Could you check a few things on this model? Use its own coordinates, in mm. Face numbers are marked on the shaded views. A direction names the side the tool comes from. Coordinates: 2 decimals unless noted, no trailing zeros. Loops run counter-clockwise (first coordinate to the right, second up) from the corner with the lowest first, then second, coordinate; pieces in that order, holes last.
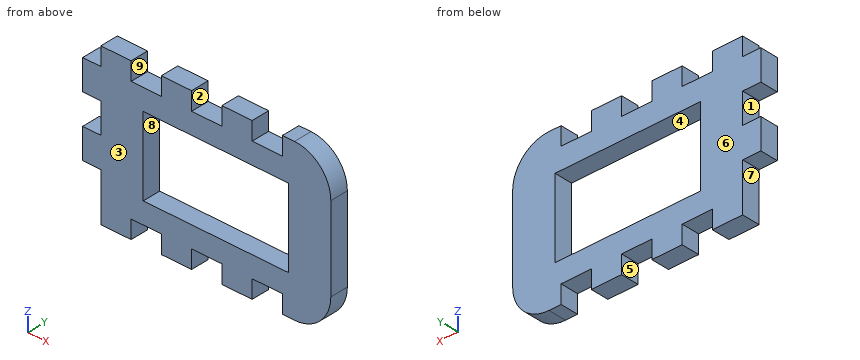
from build123d import *

# Parameters (mm, degrees)
SKETCH1_W           = 38
SKETCH1_H           = 26
BOSS_EXTRUDE1_DEPTH = 1.5
SKETCH2_W           = 24
SKETCH2_H           = 13
CUT_EXTRUDE1_DEPTH  = 3
SKETCH8_W           = 5
SKETCH8_H           = 3
BOSS_EXTRUDE2_DEPTH = 3
SKETCH9_W           = 5
SKETCH9_H           = 3
CUT_EXTRUDE2_DEPTH  = 3
FILLET1_R           = 6


with BuildPart() as part:
    # Sketch1 → Boss-Extrude1 (new body, symmetric)
    with BuildSketch(Plane(origin=(0, 0, 0), x_dir=(1, 0, 0), z_dir=(0, 1, 0))):
        Rectangle(SKETCH1_W, SKETCH1_H)
    extrude(amount=BOSS_EXTRUDE1_DEPTH, both=True)

    # Sketch2 → Cut-Extrude1 (cut)
    with BuildSketch(Plane.XZ.offset(1.5)):
        Rectangle(SKETCH2_W, SKETCH2_H)
    extrude(amount=-CUT_EXTRUDE1_DEPTH, mode=Mode.SUBTRACT)

    # Sketch8 → Boss-Extrude2 (add)
    with BuildSketch(Plane.ZY.offset(19)):
        with Locations((-2.5, 0)):
            Rectangle(SKETCH8_W, SKETCH8_H)
        with Locations((7.5, 0)):
            Rectangle(SKETCH8_W, SKETCH8_H)
    extrude(amount=BOSS_EXTRUDE2_DEPTH)

    # Sketch9 → Cut-Extrude2 (cut)
    with BuildSketch(Plane.XZ.offset(1.5)):
        with Locations((-11.5, -11.5)):
            Rectangle(SKETCH9_W, SKETCH9_H)
        with Locations((-11.5, 11.5)):
            Rectangle(SKETCH9_W, SKETCH9_H)
        with Locations((-1.5, -11.5)):
            Rectangle(SKETCH9_W, SKETCH9_H)
        with Locations((-1.5, 11.5)):
            Rectangle(SKETCH9_W, SKETCH9_H)
        with Locations((8.5, -11.5)):
            Rectangle(SKETCH9_W, SKETCH9_H)
        with Locations((8.5, 11.5)):
            Rectangle(SKETCH9_W, SKETCH9_H)
    extrude(amount=-CUT_EXTRUDE2_DEPTH, mode=Mode.SUBTRACT)

    # Fillet1
    fillet1_edges = [part.edges().sort_by_distance(p)[0] for p in [
        (19, 0, 13),
        (19, 0, -13),
    ]]
    fillet(fillet1_edges, radius=FILLET1_R)


solid = part.part
1) Imagine slicing it at A-A on z = 6. List the corners of the cut face in (x, y) for me.
2) For the marked faces 1, 2, 3, 4 and 5, which set-ups out of +Z, -Z, +X, -X, +Y, -Y let a thin tool reach every point of the face, with its end or its side?
3) If I drill on L1, parallel to X at y = 0.8, z = 1; L2, parallel to Z at x = -5, y = -0.1; L3, parallel to X at y = 0.1, z = -1.5, over which ranges is the centre line in solid material (lowest first)?
4) Will these pins go through, and if not, where does the flat tip stop? pin 1 (1 mm diameter, centred on y = -0.5, z = 8, fed in from +X); pin 2 (1.5 mm diameter, centred on y = 0.5, z = 3, fed in from -X); pin 3 (1.5 mm diameter, centred on y = 0, z = -11, fed in from +X).
5) We'd pull the mould along X, two halves only. Please class the marked faces 6, 7, 8 and 9: released by +X, released by -X, zero draft, split by the parting line, or undercut.
6) Imagine slicing it at B-B on x = 10. List the corners of the cut face in (y, z) for me.
Solved:
1. outline: (-22, -1.5) - (-12, -1.5) - (-12, 1.5) - (-22, 1.5) - close; (12, -1.5) - (19, -1.5) - (19, 1.5) - (12, 1.5) - close
2. face 1: -X, +Y, -Y
2. face 2: +Z, +Y, -Y
2. face 3: +Z, -Z, +X, -X, -Y
2. face 4: +Y, -Y
2. face 5: -Z, +Y, -Y
3. L1: x = -19 to -12, 12 to 19
3. L2: z = -13 to -6.5, 6.5 to 13
3. L3: x = -22 to -12, 12 to 19
4. pin 1: stops at x = 18.98
4. pin 2: stops at x = -19
4. pin 3: stops at x = 18.04
5. face 6: zero draft
5. face 7: released by -X
5. face 8: undercut
5. face 9: undercut
6. outline: (-1.5, -10) - (1.5, -10) - (1.5, -6.5) - (-1.5, -6.5) - close; (-1.5, 6.5) - (1.5, 6.5) - (1.5, 10) - (-1.5, 10) - close
